The model under review builds one solid part; all positions refer to its coordinate system, in mm. A direction names the side the tool comes from. Coordinates: 2 decimals unless noted, no trailing zeros. Loops run counter-clockwise (first coordinate to the right, second up) from the corner with the lowest first, then second, coordinate; pieces in that order, holes last. Notation, with made-up numbers: M 75.25,77 L 101.25,77 A29 cw 101.25,112 Z; hole C 5.25,-3 d1. An arc over 180 degrees is marked long. One line per item, written item: value.
```python
from build123d import *

# Parameters (mm, degrees)
F0_W     = 39.6
F0_H     = 28.6
F1_DEPTH = 2
F2_W     = 8
F2_H     = 4
F3_DEPTH = 20
F4_R     = 3.5
F5_DEPTH = 8
F6_R     = 3
F7_DEPTH = 6


with BuildPart() as f1:
    # F0 (on Top) → F1 (new body)
    with BuildSketch(Plane.XY):
        Rectangle(F0_W, F0_H)
    extrude(amount=F1_DEPTH)

    # F2 (on Right) → F3 (join)
    with BuildSketch(Plane.YZ):
        with Locations((-2.3, -2)):
            Rectangle(F2_W, F2_H)
    extrude(amount=-F3_DEPTH)

    # F4 (on face) → F5 (join)
    with BuildSketch(Plane.XY.offset(2)):
        with Locations((12, -1.8)):
            Circle(F4_R)
    extrude(amount=F5_DEPTH)

    # F6 (on face) → F7 (join)
    with BuildSketch(Plane.XY.offset(10)):
        with Locations((12, -1.8)):
            Circle(F6_R)
    extrude(amount=F7_DEPTH)


solid = f1.part
```
(1) Add section D-D on x = 12. State the section outline as (y, z) points.
Checks:
outline: M -14.3,0 L 14.3,0 L 14.3,2 L 1.7,2 L 1.7,10 L 1.2,10 L 1.2,16 L -4.8,16 L -4.8,10 L -5.3,10 L -5.3,2 L -14.3,2 Z
(2) Add section A-A on y = -1.8. State the section outline as (x, z) points, then the cut area to 3 significant figures.
Checks:
outline: M -20,-4 L 0,-4 L 0,0 L 19.8,0 L 19.8,2 L 15.5,2 L 15.5,10 L 15,10 L 15,16 L 9,16 L 9,10 L 8.5,10 L 8.5,2 L -19.8,2 L -19.8,0 L -20,0 Z
area: 251 mm^2
(3) Add section C-C on z = 13.5. State the section outline as (x, y) points.
Checks:
outline: C 12,-1.8 d6
(4) Insertion check: pin 1 Ø14.5 at (x, y) = (4, 2) entering from -Z; pin 2 Ø2 at (x, z) = (-9.5, -2) entering from +Y; pin 3 Ø0.6 at (y, z) = (-2, 0.5) entering from -X; pin 4 Ø4 at (x, z) = (-9.5, 5) entering from -Y. Each pin has a flat end and moves straight along its axis. Give the tip position at first contact, or say it passes through.
Checks:
pin 1: z = -4
pin 2: y = 1.7
pin 3: x = -19.8
pin 4: through
(5) Tool access review of faces 1 (the face through (-10, 1.7, -2)), 2 (the face through (0, -2, -2)), 3 (the face through (-19.8, 0, 1)): name each direction out of +Z, -Z, +X, -X, +Y, -Y from which nothing blocks a thin tool from reaching the whole face with its end or side.
Checks:
face 1: -Z, +X, -X, +Y
face 2: -Z, +X, +Y, -Y
face 3: +Z, -X, +Y, -Y
(6) To check wall thickness, follow L1, parallel to Z at x = -6.5, y = 9; L2, parallel to Z at x = -8.5, y = -5.25; L3, parallel to X at y = 1, z = 9.25. State the ranges of each line that lie inside material, in increasing order. Write a range as [from, to].
Checks:
L1: [0, 2]
L2: [-4, 2]
L3: [9.9, 14.1]
(7) Add section B-B on x = -13. State the section outline as (y, z) points.
Checks:
outline: M -14.3,0 L -6.3,0 L -6.3,-4 L 1.7,-4 L 1.7,0 L 14.3,0 L 14.3,2 L -14.3,2 Z
